The figure shows three views and two pictorial views of one solid part (mm, origin at its lowest corner). Answer the questions. Coordinates: 2 decimals unless noted, no trailing zeros. Write each loop counter-clockwise with the first axis right and the second up, starting at its lowest first coordinate (ties: lowest second). Pieces come first, ordered by that corner, then holes. Notation, with made-up numbers: (23, 65) - (77, 65) arc R13 ccw to (77, 83) - close; hole circle Ø1 at (82.25, -12). An arc over 180 degrees is marked (long way). Use a Markdown table: item, result. Add a question column.
(1) The part is cut by section B-B, the plane y = 218. Give the vertices of the cut face in (x, z).
(2) Find the intervals of material crossed by line 1 (X direction, y = 222, z = 62.5); line 2 (X direction, y = 182, z = 19), in increasing order. Write a range as from..to.
(3) The part is cut by section A-A, the plane z = 48.5. Give the vertices of the cut face in (x, y) (3 decimals).
(4) The part is cut by section C-C, the plane x = 4. Give the vertices of the cut face in (y, z), then the cut area to 3 significant figures.
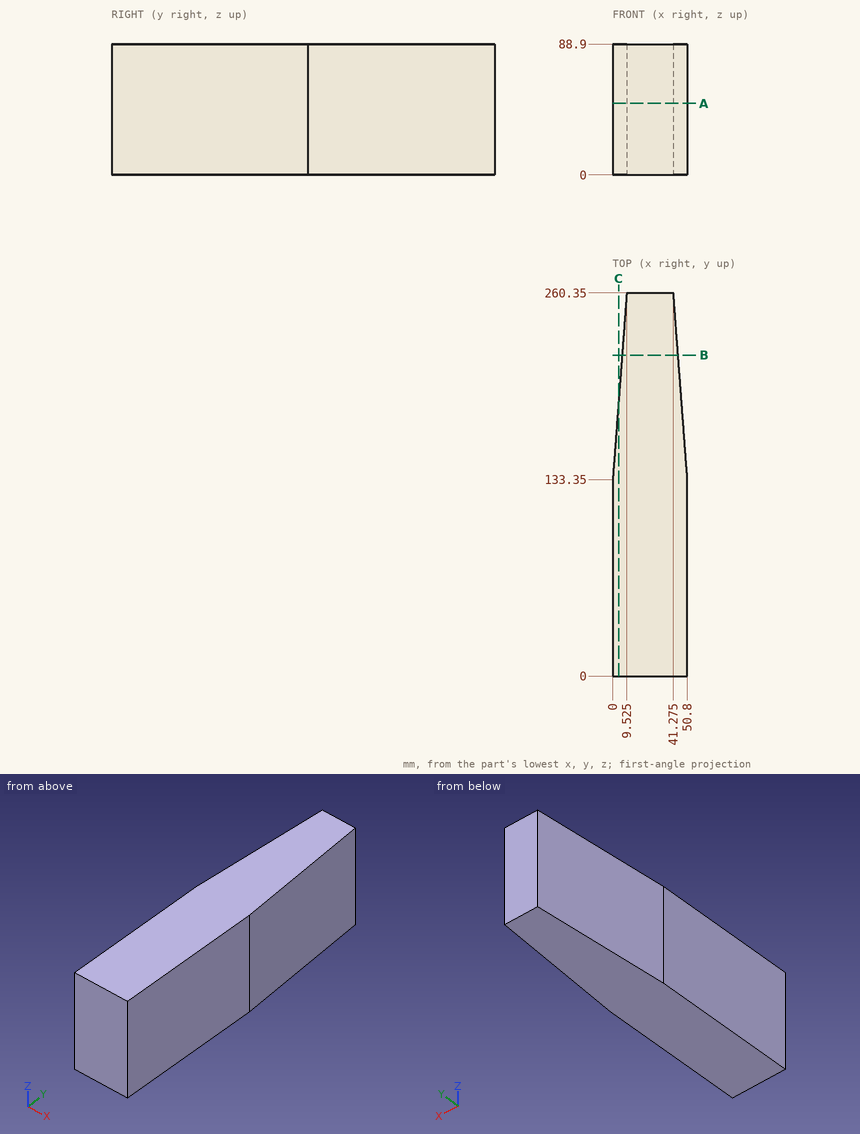
Model answer:
| question | item | result |
|---|---|---|
| 1 | outline | (6.35, 0) - (44.45, 0) - (44.45, 88.9) - (6.35, 88.9) - close |
| 2 | line 1 | 6.65..44.15 |
| 2 | line 2 | 3.65..47.15 |
| 3 | outline | (0, 0) - (50.8, 0) - (50.8, 133.35) - (41.275, 260.35) - (9.525, 260.35) - (0, 133.35) - close |
| 4 | outline | (0, 0) - (186.68, 0) - (186.68, 88.9) - (0, 88.9) - close |
| 4 | area | 16,600 mm^2 |
